from build123d import *

# Parameters (mm, degrees)
EXTRUDE_1_DEPTH          = 30
SKETCH_2_R               = 2.5
CUT_EXTRUDE_1_DEPTH      = 21
CUT_EXTRUDE_2_DEPTH      = 1
CUT_EXTRUDE_2_DEPTH_BACK = 47


with BuildPart() as part:
    # Эскиз1 → Бобышка-Вытянуть1 (new body)
    with BuildSketch(Plane(origin=(0, 0, 0), x_dir=(1, 0, 0), z_dir=(0, 1, 0))):
        Polygon((0, 0), (0, -90), (-30, -90), (-30, 20), (16, 20), (16, 0), align=None)
    extrude(amount=EXTRUDE_1_DEPTH)

    # Эскиз2 → Вырез-Вытянуть1 (cut, through all)
    with BuildSketch(Plane.XY):
        with Locations((6, 15)):
            Circle(SKETCH_2_R)
    extrude(amount=-CUT_EXTRUDE_1_DEPTH, mode=Mode.SUBTRACT)

    # Эскиз3 → Вырез-Вытянуть2 (cut, two sides)
    with BuildSketch(Plane.ZY.offset(30)) as cut_extrude_2_sk:
        Polygon((323.973212684, 21), (90, 21), (80, 21), (80, 9), (90, 9), (323.973212684, 9), (791.919638052, 9), (791.919638052, 21), align=None)
    extrude(amount=CUT_EXTRUDE_2_DEPTH, mode=Mode.SUBTRACT)
    extrude(cut_extrude_2_sk.sketch, amount=-CUT_EXTRUDE_2_DEPTH_BACK, mode=Mode.SUBTRACT)


solid = part.part
Work out the finished part from the listing and answer in its coordinate system (mm). A direction names the side the tool comes from. Give positions to 0.01 mm unless a question says otherwise; leave off trailing zeros. Write each loop counter-clockwise with the first axis right and the second up, starting at its lowest first coordinate (ties: lowest second). Pieces come first, ordered by that corner, then holes.
Q1. The part is cut by section D-D on x = -11.5. Give the vertices of the cut face in (y, z).
Answer:
outline: (0, -20) - (30, -20) - (30, 90) - (21, 90) - (21, 80) - (9, 80) - (9, 90) - (0, 90) - close
Q2. Straight lines are drawn through the part: L1, parallel to Y at x = 6, z = -12; L2, parallel to Z at x = -24, y = 14.5; L3, parallel to Z at x = 5, y = 18.5. For each, find the intervals that lie inside material, in ascending order.
Answer:
L1: y = 0 to 12.5, 17.5 to 30
L2: z = -20 to 80
L3: z = -20 to 0
Q3. The part is cut by section C-C on y = 10.5. Give the vertices of the cut face in (x, z).
Answer:
outline: (-30, -20) - (16, -20) - (16, 0) - (0, 0) - (0, 80) - (-30, 80) - close
Q4. For a pull along Y with two mould halves and no side action, classify faces 1 (the face through (-12, 30, 34)), 2 (the face through (16, 15, -10)), 3 (the face through (-15, 15, 80)) as released by +Y, released by -Y, zero draft, split by the parting line, or undercut.
Answer:
face 1: released by +Y
face 2: zero draft
face 3: undercut
Q5. Given pin 1 (1.5 mm diameter, centred on y = 13, z = 42, fed in from +X); pin 2 (8 mm diameter, centred on x = 5, y = 11.5, fed in from +Z); pin 3 (6 mm diameter, centred on x = -14.5, y = 14, fed in from +Z), each flat-ended and moving along its own axis, determine where each tip first touches the part or whether it passes through.
Answer:
pin 1: stops at x = 0
pin 2: stops at z = 0
pin 3: stops at z = 80
Q6. The part is cut by section A-A on y = 15. Give the vertices of the cut face in (x, z), and give its area (3 significant figures).
Answer:
outline: (-30, -20) - (3.5, -20) - (3.5, 0) - (0, 0) - (0, 80) - (-30, 80) - close; (8.5, -20) - (16, -20) - (16, 0) - (8.5, 0) - close
area: 3,220 mm2
Q7. A tool of negligible diameter and unlimited length cuts with its end or side. For faces 4 (the face through (10, 15, 0)), 5 (the face through (-15, 21, 85)), 6 (the face through (-15, 4, 90)), from which of +Z, -Z, +X, -X, +Y, -Y can it reach the whole face along a straight path? Write none if from no direction.
Answer:
face 4: +Z, +X, +Y, -Y
face 5: +Z, +X, -X
face 6: +Z, +X, -X, +Y, -Y
Q8. The part is cut by section B-B on x = 6. Give the vertices of the cut face in (y, z).
Answer:
outline: (0, -20) - (12.5, -20) - (12.5, 0) - (0, 0) - close; (17.5, -20) - (30, -20) - (30, 0) - (17.5, 0) - close
